Check sheet for the modelled part. Datum: model origin and axes. Units: mm. Round coordinates to 2 decimals unless told otherwise and drop trailing zeros. Write each loop counter-clockwise with the first axis right and the second up, starting at its lowest first coordinate (ties: lowest second). Pieces come first, ordered by that corner, then holes. Notation, with made-up numbers: (48, 47) - (56, 47) arc R28 ccw to (56, 84) - close; hole circle Ø7 at (83.5, 31.25). An arc over 180 degrees is marked (long way). Answer as a JSON object with one key per item and string values. Group by question number.
Item 1: Sectioned sample at C-C on y = 156. Record the boundary of the cut face in (x, z).
Item 2: Thickness scan on line 1 (Y direction, x = 2.5, z = 3); line 2 (Z direction, x = -4, y = 90); line 3 (Z direction, x = -11.5, y = 100). Record the ranges inside material, lowest first.
Item 3: Release check for a two-part mould opening along X. For faces 1 (the cylindrical face through (4.71, 161.27, 39.86)), 2 (the cylindrical face through (4.71, 8.73, 39.86)), 3 (the flat face through (-5, 17.7, 12)), 4 (the flat face through (-34.784, 9, -4)) record: pulls with the +X half, pulls with the -X half, needs draft (parallel to the pull), parting line crosses it, or undercut.
Item 4: Sectioned sample at B-B on x = -3.5. Record the boundary of the cut face in (y, z).
Item 5: Gauge pin test, flat ends, axial feed: P1, Ø1, axis at y = 95, z = -42, coming from the +X side; P2, Ø3, axis at y = 23.5, z = -33.5, coming from the -X side; P3, Ø12, axis at x = -1, y = 54.5, coming from the -Z side. Record the tip position at first contact, or that the pin passes through.
Item 6: Sectioned sample at D-D on z = 37.5. Record the boundary of the cut face in (x, y), plus the area to 3 significant figures.
Item 7: Sectioned sample at A-A on z = 3.5. Record the boundary of the cut face in (x, y).
```python
from build123d import *

# Parameters (mm, degrees)
F0_R     = 9.296247
F1_DEPTH = 85
F0_R_2   = 10.278889
F2_DEPTH = 17.7


with BuildPart() as f1:
    # F0 (on Front) → F1 (new body)
    with BuildSketch(Plane.XZ):
        with BuildLine():
            ThreePointArc((25.215676, -48.521861), (-4.784324, -18.521861), (-34.784324, -48.521861))
            ThreePointArc((-34.784324, -48.521861), (-4.784324, -78.521861), (25.215676, -48.521861))
        make_face()
        with Locations((-4.784324, -48.521861)):
            Circle(F0_R, mode=Mode.SUBTRACT)
    extrude(amount=-F1_DEPTH)

    # F0 (on Front) → F2 (join)
    with BuildSketch(Plane.XZ):
        with BuildLine():
            ThreePointArc((25.215676, 40.099124), (-4.784324, 70.099124), (-34.784324, 40.099124))
            Line((-34.784324, 40.099124), (-34.784324, -48.521861))
            ThreePointArc((-34.784324, -48.521861), (-4.784324, -18.521861), (25.215676, -48.521861))
            Line((25.215676, -48.521861), (25.215676, 40.099124))
        make_face()
        with Locations((-4.784844, 43.795345)):
            Circle(F0_R_2, mode=Mode.SUBTRACT)
        with BuildLine():
            ThreePointArc((25.215676, -48.521861), (-4.784324, -18.521861), (-34.784324, -48.521861))
            ThreePointArc((-34.784324, -48.521861), (-4.784324, -78.521861), (25.215676, -48.521861))
        make_face()
        with Locations((-4.784324, -48.521861)):
            Circle(F0_R, mode=Mode.SUBTRACT)
    extrude(amount=-F2_DEPTH)

    # F4: F1 across plane


with BuildPart() as f1_1:
    add(f1.part)
    add(f1.part.mirror(Plane.XZ.offset(-85)))


solid = f1_1.part
```
Completed:
{
 "1": {"outline": "(-34.78, -48.52) arc R30 ccw to (25.22, -48.52) - (25.22, 40.1) arc R30 ccw to (-34.78, 40.1) - close; hole circle Ø20.56 at (-4.78, 43.8); hole circle Ø18.59 at (-4.78, -48.52)"},
 "2": {"line 1": "0 to 17.7, 152.3 to 170", "line 2": "-78.51 to -57.78, -39.26 to -18.53", "line 3": "-77.76 to -54.95, -42.09 to -19.28"},
 "3": {"face 1": "undercut", "face 2": "undercut", "face 3": "needs draft", "face 4": "pulls with the -X half"},
 "4": {"outline": "(0, -78.49) - (170, -78.49) - (170, -57.73) - (0, -57.73) - close; (0, -39.31) - (170, -39.31) - (170, 33.6) - (152.3, 33.6) - (152.3, -18.55) - (17.7, -18.55) - (17.7, 33.6) - (0, 33.6) - close; (0, 53.99) - (17.7, 53.99) - (17.7, 70.07) - (0, 70.07) - close; (152.3, 53.99) - (170, 53.99) - (170, 70.07) - (152.3, 70.07) - close"},
 "5": {"P1": "x = 24.61", "P2": "x = -31.56", "P3": "z = -78.52"},
 "6": {"outline": "(-34.78, 0) - (-12.91, 0) - (-12.91, 17.7) - (-34.78, 17.7) - close; (-34.78, 152.3) - (-12.91, 152.3) - (-12.91, 170) - (-34.78, 170) - close; (3.34, 0) - (25.22, 0) - (25.22, 17.7) - (3.34, 17.7) - close; (3.34, 152.3) - (25.22, 152.3) - (25.22, 170) - (3.34, 170) - close", "area": "1,550 mm²"},
 "7": {"outline": "(-34.78, 0) - (25.22, 0) - (25.22, 17.7) - (-34.78, 17.7) - close; (-34.78, 152.3) - (25.22, 152.3) - (25.22, 170) - (-34.78, 170) - close"}
}
